Read the model definition and answer for the solid it produces. Units are mm, in the model's axes. Face numbers are marked on the shaded views. Give positions to 0.01 mm unless a question says otherwise; leave off trailing zeros. Order: outer loops, then holes, each group sorted by start corner. A loop starts at its lowest first (then second) coordinate and runs counter-clockwise, first axis right, second up. Notation, with made-up numbers: (-29, 13.25) - (-15, 13.25) arc R25 cw to (-15, 50.25) - close; hole circle Ø4 at (-17.75, -9). An arc over 180 degrees is marked (long way). Write each question's results on one line, items separated by ' | '.
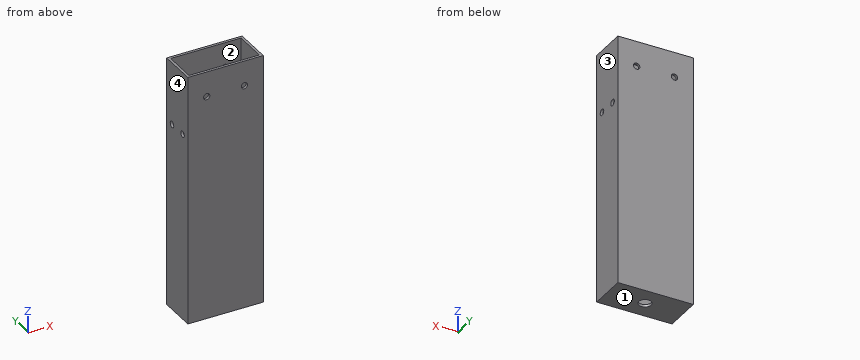
from build123d import *

# Parameters (mm, degrees)
F0_W       = 76.2
F0_H       = 38.1
F1_DEPTH   = 254
F2_T       = -2.54
F5_D       = 6.35
F5_ON_F4_D = 6.35
F7_D       = 12.7


with BuildPart() as f1:
    # F0 (on Top) → F1 (new body)
    with BuildSketch(Plane.XY):
        Rectangle(F0_W, F0_H)
    extrude(amount=F1_DEPTH)

    # F2
    f2_openings = [f1.faces().sort_by_distance(p)[0] for p in [
        (0, 0, 254),
    ]]
    offset(amount=F2_T, openings=f2_openings)

    # F5 (through all)
    with Locations(Plane(origin=(-38.1, 0, 0), x_dir=(0, -1, 0), z_dir=(-1, 0, 0))):
        with Locations((-9.525, 190.5), (9.525, 190.5)):
            Hole(F5_D / 2)

    # F5 on F4 (through all)
    with Locations(Plane.XZ.offset(19.05)):
        with Locations((-19.05, 228.6), (19.05, 228.6)):
            Hole(F5_ON_F4_D / 2)

    # F7 (through all)
    with Locations(Plane(origin=(0, 0, 0), x_dir=(1, 0, 0), z_dir=(0, 0, -1))):
        with Locations((0, 0)):
            Hole(F7_D / 2)


solid = f1.part
(1) Each of these flat-tipped pins is pushed along its axis until it touches: pin 1 (4 mm diameter, centred on y = -9.525, z = 190.5, fed in from -X); pin 2 (7.5 mm diameter, centred on y = -9.525, z = 190.5, fed in from -X); pin 3 (12 mm diameter, centred on x = 28, y = 6, fed in from +Z). Where does it stop, or does it pass through?
Conclusion:
pin 1: through | pin 2: x = -38.1 | pin 3: z = 2.54
(2) Section A-A (y = 0) is taken. Give the vertices of the cut face in (x, z), plus the area to 3 significant figures.
Conclusion:
outline: (-38.1, 0) - (-6.35, 0) - (-6.35, 2.54) - (-35.56, 2.54) - (-35.56, 254) - (-38.1, 254) - close; (6.35, 0) - (38.1, 0) - (38.1, 254) - (35.56, 254) - (35.56, 2.54) - (6.35, 2.54) - close | area: 1,440 mm^2
(3) Section C-C (z = 219.5) is taken. Give the vertices of the cut face in (x, y), plus the area to 3 significant figures.
Conclusion:
outline: (-38.1, -19.05) - (38.1, -19.05) - (38.1, 19.05) - (-38.1, 19.05) - close; hole (-35.56, -16.51) - (35.56, -16.51) - (35.56, 16.51) - (-35.56, 16.51) - close | area: 555 mm^2
(4) Consider probe 1 along Y at (x, z) = (36, 190); probe 2 along X at (y, z) = (-17.4, 228.6) (3 decimals); probe 3 along X at (y, z) = (-1, 229). Determine where each line is inside the solid, lowest interval first. Write a range as [from, to].
Conclusion:
probe 1: [-19.05, -12.66], [-6.39, 6.39], [12.66, 19.05] | probe 2: [-38.1, -22.225], [-15.875, 15.875], [22.225, 38.1] | probe 3: [-38.1, -35.56], [35.56, 38.1]
(5) Section D-D (x = 0) is taken. Give the vertices of the cut face in (y, z), plus the area to 3 significant figures.
Conclusion:
outline: (-19.05, 0) - (-6.35, 0) - (-6.35, 2.54) - (-16.51, 2.54) - (-16.51, 254) - (-19.05, 254) - close; (6.35, 0) - (19.05, 0) - (19.05, 254) - (16.51, 254) - (16.51, 2.54) - (6.35, 2.54) - close | area: 1,340 mm^2
(6) The mould has two halves that part along X. Classify the marked faces 1, 2, 3 and 4: pulls with the +X half, pulls with the -X half, needs draft (parallel to the pull), parting line crosses it, or undercut.
Conclusion:
face 1: needs draft | face 2: undercut | face 3: pulls with the +X half | face 4: pulls with the -X half
(7) Section B-B (x = 19.05) is taken. Give the vertices of the cut face in (y, z) (3 decimals).
Conclusion:
outline: (-19.05, 0) - (19.05, 0) - (19.05, 225.425) - (16.51, 225.425) - (16.51, 2.54) - (-16.51, 2.54) - (-16.51, 225.425) - (-19.05, 225.425) - close; (-19.05, 231.775) - (-16.51, 231.775) - (-16.51, 254) - (-19.05, 254) - close; (16.51, 231.775) - (19.05, 231.775) - (19.05, 254) - (16.51, 254) - close
